Autodesk Inventor part; units mm, degrees
ref_plane "YZ Plane" through (0, 0, 0) normal (1, 0, 0) x (0, 1, 0)
ref_plane "XZ Plane" through (0, 0, 0) normal (0, 1, 0) x (-1, 0, 0)
ref_plane "XY Plane" through (0, 0, 0) normal (0, 0, 1) x (1, 0, 0)
sketch "Sketch1" plane through (0, 0, 0) normal (0, 1, 0) x (-1, 0, 0)
  line L0 (0, 0) -> (0, -25.4)
  line L1 (0, -25.4) -> (3.175, -25.4)
  line L2 (3.175, -25.4) -> (3.175, -3.175)
  line L3 (3.175, -3.175) -> (25.4, -3.175)
  line L4 (25.4, -3.175) -> (25.4, 0)
  line L5 (25.4, 0) -> (0, 0)
  dimension "d0" = 25.4
  dimension "d1" = 3.175
  dimension "d2" = 22.225
  dimension "d3" = 22.225
extrude "Extrusion1" add sketch "Sketch1" along normal blind 63.5
sketch "Sketch2" plane through (-25.4, 0, 0) normal (0, 0, 1) x (1, 0, 0)
  line L0 (22.225, 0) -> (22.225, 63.5)
  line L1 (22.225, 0) -> (15.875, 0)
  line L2 (22.225, 0) -> (0, 0)
  line L3 (22.225, 63.5) -> (0, 63.5)
  circle A0 centre (15.875, 57.15) radius 3.81
  circle A1 centre (15.875, 6.35) radius 3.81
  circle A2 centre (-9.525, 31.75) radius 24.13
  line L4 (22.225, 31.75) -> (-9.525, 31.75)
  point P0 (25.4, 0)
  dimension "d6" = 6.35
  dimension "d9" = 7.62
  dimension "d10" = 7.62
  dimension "d12" = 31.75
extrude "Extrusion2" cut sketch "Sketch2" against normal blind 63.5
sketch "Sketch3" plane through (0, 0, 0) normal (1, 0, 0) x (0, 0, -1)
  line L0 (25.4, 0) -> (25.4, 63.5)
  circle A0 centre (12.7, 12.7) radius 3.81
  line L1 (0, 9.5795) -> (0, 53.9205)
  circle A1 centre (12.7, 50.8) radius 3.81
  point P0 (0, 0)
extrude "Extrusion3" cut sketch "Sketch3" against normal blind 63.5
properties part number "Bracket"
Model file for the job. Use its own axes, mm. A direction names the side the tool comes from. Round coordinates to 2 decimals unless told otherwise and drop trailing zeros. Order: outer loops, then holes, each group sorted by start corner. A loop starts at its lowest first (then second) coordinate and runs counter-clockwise, first axis right, second up.
(1) Pin check, flat tips, straight feed: pin 1 (4.5 mm diameter, centred on x = -9.525, y = 57.15, fed in from -Z); pin 2 (11 mm diameter, centred on y = 26, z = -13.5, fed in from -X) (3 decimals). Stop position of each tip, or through.
(2) Drill centre lines: line 1 (Y direction, x = -2, z = -12.7); line 2 (X direction, y = 29, z = -21.5) (3 decimals). Where is each one in solid material? Low to high.
(3) Band-saw the part on A-A (z = -12.7). List the corners of the cut face in (x, y) (3 decimals).
(4) Band-saw the part on C-C (x = -19.25). List the corners of the cut face in (y, z) (3 decimals), then the cut area to 3 significant figures.
(5) Band-saw the part on B-B (y = 6.35). List the corners of the cut face in (x, z) (3 decimals), then the cut area to 3 significant figures.
(6) Band-saw the part on D-D (x = -8.5). List the corners of the cut face in (y, z) (3 decimals).
(7) Pull direction Y, two halves, no side cores. Call faces 3 (the face through (-1.57, 10.38, -9.68)), 4 (the face through (-2, 63.5, -7)), 5 (the face through (-1.565, 54.578, -12.204)), 6 (the face through (-9, 31, -3.175)): released by +Y, released by -Y, zero draft, split by the parting line, or undercut.
(8) 3-axis set-ups, long thin cutter, end or side, ignore diameter. For faces 1 (the face through (-25.4, 5, -2)), 2 (the face through (-3.175, 31, -14)): which of +Z, -Z, +X, -X, +Y, -Y reach the whole face in a straight line?
Verdict:
1. pin 1: passes through
1. pin 2: stops at x = -3.175
2. line 1: y = 0 to 8.89, 16.51 to 46.99, 54.61 to 63.5
2. line 2: x = -3.175 to 0
3. outline: (-3.175, 0) - (0, 0) - (0, 8.89) - (-3.175, 8.89) - close; (-3.175, 16.51) - (0, 16.51) - (0, 46.99) - (-3.175, 46.99) - close; (-3.175, 54.61) - (0, 54.61) - (0, 63.5) - (-3.175, 63.5) - close
4. outline: (0, -3.175) - (13.405, -3.175) - (13.405, 0) - (0, 0) - close; (50.095, -3.175) - (63.5, -3.175) - (63.5, 0) - (50.095, 0) - close
4. area: 85.1 mm2
5. outline: (-25.4, -3.175) - (-13.335, -3.175) - (-13.335, 0) - (-25.4, 0) - close; (-5.715, -3.175) - (-3.175, -3.175) - (-3.175, -25.4) - (0, -25.4) - (0, 0) - (-5.715, 0) - close
5. area: 127 mm2
6. outline: (0, -3.175) - (2.68, -3.175) - (2.68, 0) - (0, 0) - close; (10.02, -3.175) - (53.48, -3.175) - (53.48, 0) - (10.02, 0) - close; (60.82, -3.175) - (63.5, -3.175) - (63.5, 0) - (60.82, 0) - close
7. face 3: undercut
7. face 4: released by +Y
7. face 5: undercut
7. face 6: zero draft
8. face 1: +Z, -Z, -X, +Y, -Y
8. face 2: -Z, -X, +Y, -Y
